Build history of the part. All positions in model axes, mm. Round coordinates to 2 decimals unless told otherwise and drop trailing zeros. Loops run counter-clockwise (first coordinate to the right, second up) from the corner with the lowest first, then second, coordinate; pieces in that order, holes last. Notation, with made-up numbers: (64, -10.75) - (120, -10.75) arc R33 cw to (120, 18.25) - close; hole circle Ø8 at (59, 78.25). An arc over 180 degrees is marked (long way). Use a Markdown table: item, result.
from build123d import *

# Parameters (mm, degrees)
SKETCH1_W           = 320
SKETCH1_H           = 200
BOSS_EXTRUDE1_DEPTH = 15.875
FILLET1_R           = 160
FILLET2_R           = 10
SKETCH2_R           = 13
CUT_EXTRUDE1_DEPTH  = 190.346284952
SKETCH3_R           = 2.5
CUT_EXTRUDE2_DEPTH  = 190.346284952
SKETCH4_R           = 2.5
CUT_EXTRUDE3_DEPTH  = 190.346284952
SKETCH5_R           = 1.5625
CUT_EXTRUDE4_DEPTH  = 190.346284952


with BuildPart() as part:
    # Sketch1 → Boss-Extrude1 (new body)
    with BuildSketch(Plane.XY):
        Rectangle(SKETCH1_W, SKETCH1_H)
    extrude(amount=BOSS_EXTRUDE1_DEPTH)

    # Fillet1
    fillet1_edges = [part.edges().sort_by_distance(p)[0] for p in [
        (-160, 100, 7.9375),
        (160, 100, 7.9375),
    ]]
    fillet(fillet1_edges, radius=FILLET1_R - 0.0001)  # a hair under: the kernel refuses the full size

    # Fillet2
    fillet2_edges = [part.edges().sort_by_distance(p)[0] for p in [
        (160, -100, 7.9375),
        (-160, -100, 7.9375),
    ]]
    fillet(fillet2_edges, radius=FILLET2_R)

    # Sketch2 → Cut-Extrude1 (cut, through all)
    with BuildSketch(Plane.XY.offset(15.875)):
        with Locations((0, -60)):
            Circle(SKETCH2_R)
        with Locations((0, -20)):
            Circle(SKETCH2_R)
    extrude(amount=-CUT_EXTRUDE1_DEPTH, mode=Mode.SUBTRACT)

    # Sketch3 → Cut-Extrude2 (cut, through all)
    with BuildSketch(Plane.XY.offset(15.875)):
        with Locations((-15, -5)):
            Circle(SKETCH3_R)
        with Locations((-15, -35)):
            Circle(SKETCH3_R)
        with Locations((15, -35)):
            Circle(SKETCH3_R)
        with Locations((15, -5)):
            Circle(SKETCH3_R)
    extrude(amount=-CUT_EXTRUDE2_DEPTH, mode=Mode.SUBTRACT)

    # Sketch4 → Cut-Extrude3 (cut, through all)
    with BuildSketch(Plane.XY.offset(15.875)):
        with Locations((-100, 25)):
            Circle(SKETCH4_R)
        with Locations((100, 25)):
            Circle(SKETCH4_R)
        with Locations((125, -80)):
            Circle(SKETCH4_R)
        with Locations((-125, -80)):
            Circle(SKETCH4_R)
    extrude(amount=-CUT_EXTRUDE3_DEPTH, mode=Mode.SUBTRACT)

    # Sketch5 → Cut-Extrude4 (cut, through all)
    with BuildSketch(Plane(origin=(0, 0, 0), x_dir=(-1, 0, 0), z_dir=(0, 0, -1))):
        with Locations((96.5, -51)):
            Circle(SKETCH5_R)
        with Locations((96.5, -69)):
            Circle(SKETCH5_R)
        with Locations((-96.5, -51)):
            Circle(SKETCH5_R)
        with Locations((-96.5, -69)):
            Circle(SKETCH5_R)
    extrude(amount=-CUT_EXTRUDE4_DEPTH, mode=Mode.SUBTRACT)


solid = part.part
Q1. Cut at D-D, the plane x = 69.5. List the corners of the cut face in (y, z) (3 decimals), plus the area to 3 significant figures.
Results found:
| item | result |
|---|---|
| outline | (-100, 0) - (84.117, 0) - (84.117, 15.875) - (-100, 15.875) - close |
| area | 2,920 mm2 |
Q2. Cut at A-A, the plane z = 11.5. Count the separate pieces of the cut face and the enclosed holes in it, plus the area to 3 significant figures.
Results found:
| item | result |
|---|---|
| separate pieces | 1 |
| enclosed holes | 14 |
| area | 51,700 mm2 |
Q3. Cut at C-C, the plane x = 4. List the corners of the cut face in (y, z) (3 decimals), plus the area to 3 significant figures.
Results found:
| item | result |
|---|---|
| outline | (-100, 0) - (-72.369, 0) - (-72.369, 15.875) - (-100, 15.875) - close; (-47.631, 0) - (-32.369, 0) - (-32.369, 15.875) - (-47.631, 15.875) - close; (-7.631, 0) - (99.95, 0) - (99.95, 15.875) - (-7.631, 15.875) - close |
| area | 2,390 mm2 |
Q4. Probe line 1 (Y direction, x = 96.5, z = 12.5); line 2 (Y direction, x = -15, z = 4.75); line 3 (X direction, y = -69, z = 8.5). List the from-to ranges inside material, lowest first.
Results found:
| item | result |
|---|---|
| line 1 | y = -100 to -70.56, -67.44 to -52.56, -49.44 to 67.62 |
| line 2 | y = -100 to -37.5, -32.5 to -7.5, -2.5 to 99.3 |
| line 3 | x = -160 to -98.06, -94.94 to -9.38, 9.38 to 94.94, 98.06 to 160 |
Q5. Pull direction X, two halves, no side cores. Call faces 1 (the face through (-2, -100, 8)), 2 (the face through (-2.82, -32.69, 8.05)), 3 (the face through (-1.69, -47.11, 8.05)), 4 (the face through (160, -75, 8)): pulls with the +X half, pulls with the -X half, needs draft (parallel to the pull), parting line crosses it, or undercut.
Results found:
| item | result |
|---|---|
| face 1 | needs draft |
| face 2 | undercut |
| face 3 | undercut |
| face 4 | pulls with the +X half |
Q6. Drop flat-ended pins along their axis: pin 1 (6 mm diameter, centred on y = -5.5, z = 9.5, fed in from -X); pin 2 (8 mm diameter, centred on y = 75, z = 2.5, fed in from +X); pin 3 (2 mm diameter, centred on y = 55, z = 10, fed in from -X). Give the stop position or say it passes through.
Results found:
| item | result |
|---|---|
| pin 1 | stops at x = -151.49 |
| pin 2 | stops at x = 91.86 |
| pin 3 | stops at x = -112.27 |
Q7. Cut at B-B, the plane y = -20. List the corners of the cut face in (x, z) (3 decimals).
Results found:
| item | result |
|---|---|
| outline | (-154.919, 0) - (-13, 0) - (-13, 15.875) - (-154.919, 15.875) - close; (13, 0) - (154.919, 0) - (154.919, 15.875) - (13, 15.875) - close |
